The drawing under review shows one solid part. Ordinate dimensions are in mm from its lowest x, y, z. A direction names the side the tool comes from. Give positions to 0.01 mm unless a question says otherwise; leave off trailing zeros. Write each loop counter-clockwise with the first axis right and the second up, starting at its lowest first coordinate (ties: lowest second). Pieces come first, ordered by that corner, then holes. Notation, with made-up numbers: (79, 47) - (87, 47) arc R10 cw to (87, 55) - close; hole circle Ø5 at (77.25, 24). An arc over 180 degrees is marked (long way). Write item = value, one per line.
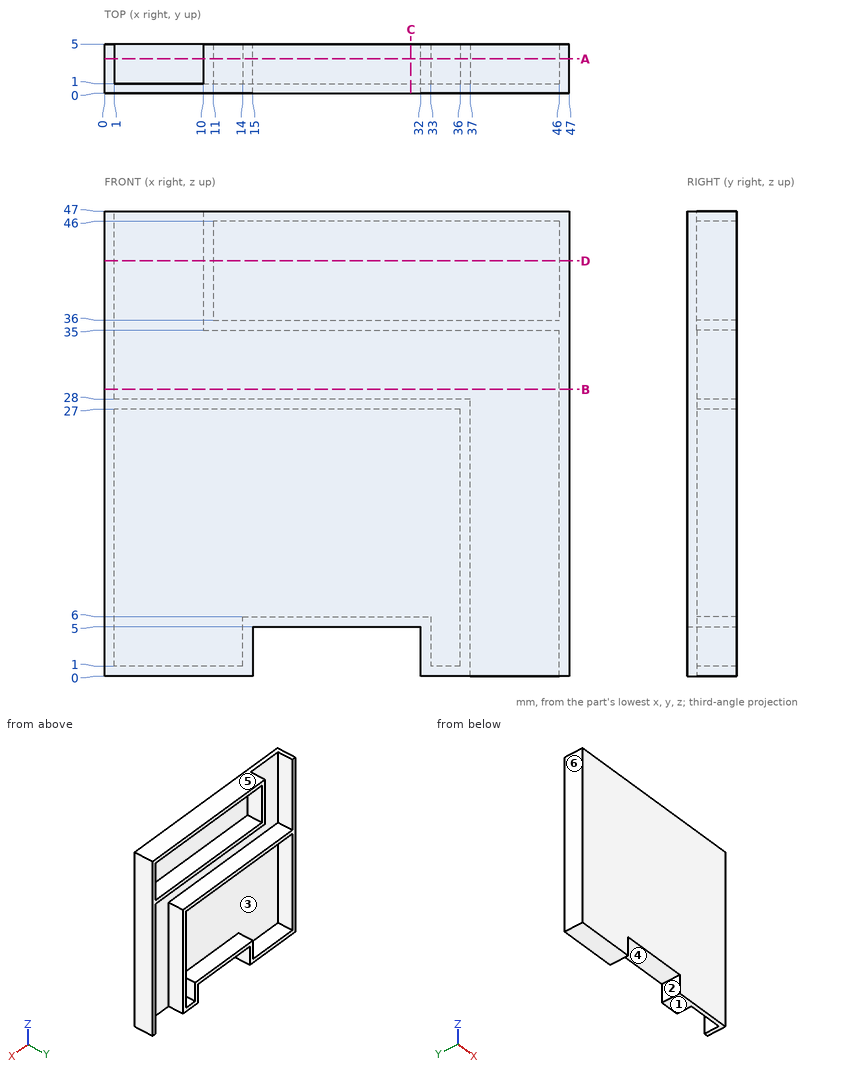
1. Draft analysis for pull direction X (two halves, no side actions). For the marked faces 3, 4, 5 and 6, state which applies: +X half, -X half, draft (parallel to the pull), parting line (faces both ways), or undercut.
Findings below:
face_3 = undercut
face_4 = undercut
face_5 = draft
face_6 = -X half
2. For line 1 (Z direction, x = 27.5, y = 2.8); line 2 (Z direction, x = 11.5, y = 1.85); line 3 (X direction, y = 3.95, z = 12), list the stretches that pass through material, from the lowest coordinate up. Write a range as from..to.
Findings below:
line_1 = 5..6, 27..28, 35..36, 46..47
line_2 = 0..1, 27..28, 35..36, 46..47
line_3 = 0..1, 36..37, 46..47
3. Insertion check: P1, Ø13, axis at x = 24.5, z = 16.5, coming from the +Y side; P2, Ø3, axis at x = 20, y = 2.5, coming from the -Z side. Each pin has a flat end and moves straight along its axis. Give the tip position at first contact, or say it passes through.
Findings below:
P1 = 1
P2 = 5
4. Take a section at B-B on z = 29. Give the boundary of the cut face in (x, y), and give its area (3 significant figures).
Findings below:
outline = (0, 0) - (47, 0) - (47, 5) - (46, 5) - (46, 1) - (1, 1) - (1, 5) - (0, 5) - close
area = 55.0 mm²
5. Take a section at C-C on x = 31. Give the boundary of the cut face in (y, z).
Findings below:
outline = (0, 5) - (5, 5) - (5, 6) - (1, 6) - (1, 27) - (5, 27) - (5, 28) - (1, 28) - (1, 35) - (5, 35) - (5, 36) - (1, 36) - (1, 46) - (5, 46) - (5, 47) - (0, 47) - close
6. Machinability: for the marked faces 1 and 2, which of the approach directions +Z, -Z, +X, -X, +Y, -Y give a long, thin tool a straight path to every point of the face, cutting with its end or side? Answer none if there is none.
Findings below:
face_1 = -Z, +X, -X, +Y, -Y
face_2 = -Z, +Y, -Y
7. Take a section at D-D on z = 42. Give the boundary of the cut face in (x, y), and give its area (3 significant figures).
Findings below:
outline = (0, 0) - (47, 0) - (47, 5) - (46, 5) - (46, 1) - (11, 1) - (11, 5) - (10, 5) - (10, 1) - (1, 1) - (1, 5) - (0, 5) - close
area = 59.0 mm²
8. Take a section at A-A on y = 3.5. Give the boundary of the cut face in (x, z).
Findings below:
outline = (0, 0) - (15, 0) - (15, 5) - (32, 5) - (32, 0) - (37, 0) - (37, 28) - (1, 28) - (1, 47) - (0, 47) - close; (10, 35) - (46, 35) - (46, 0) - (47, 0) - (47, 47) - (10, 47) - close; hole (1, 1) - (14, 1) - (14, 6) - (33, 6) - (33, 1) - (36, 1) - (36, 27) - (1, 27) - close; hole (11, 36) - (46, 36) - (46, 46) - (11, 46) - close
